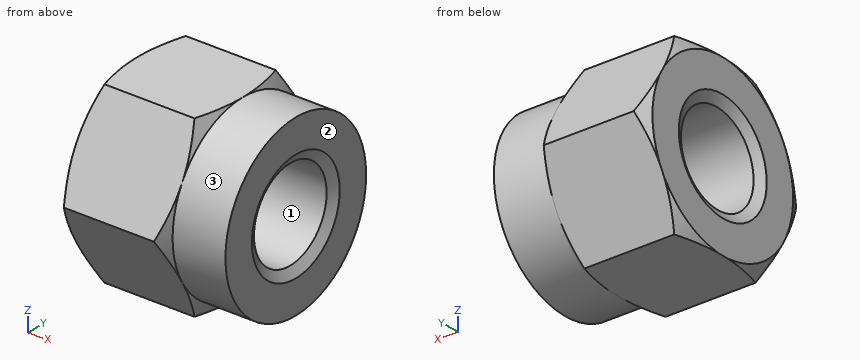
Autodesk Inventor part; units mm, degrees
ref_plane "Work Plane1" through (14.1836, 0, 0) normal (0, 0, 1) x (-1, 0, 0)
ref_plane "YZ Plane" through (0, 0, 0) normal (1, 0, 0) x (0, 1, 0)
ref_plane "XZ Plane" through (0, 0, 0) normal (0, 1, 0) x (-1, 0, 0)
sketch "Sketch1" plane through (0, 0, 0) normal (1, 0, 0) x (0, 1, 0)
  line L0 (2.3094, -4) -> (-2.3094, -4)
  line L1 (-2.3094, -4) -> (-4.6188, 0)
  line L2 (-4.6188, 0) -> (-2.3094, 4)
  line L3 (-2.3094, 4) -> (2.3094, 4)
  line L4 (2.3094, 4) -> (4.6188, 0)
  line L5 (4.6188, 0) -> (2.3094, -4)
  point P0 (0, 0)
  point P1 (0, 0)
  dimension "d0" = 9.2376
extrude "Body" add sketch "Sketch1" along normal blind 4.8
sketch "Sketch2" plane through (4.8, 0, 0) normal (1, 0, 0) x (0, 0, -1)
  circle A0 centre (0, 0) radius 4
  dimension "d7" = 8
extrude "Ring" add sketch "Sketch2" along normal blind 2.4
sketch "Sketch3" plane through (0, 0, 0) normal (0, 0, 1) x (1, 0, 0)
  line L0 (0, 2.3094) -> (0, 4.6188)
  line L1 (0, 4.6188) -> (4.8, 4.6188)
  line L2 (4.8, 2.3094) -> (4.8, 4.6188)
  line L3 (-0.96, 0) -> (5.76, 0)
  line L4 (0, 4) -> (0.3573, 4.6188)
  line L5 (4.4427, 4.6188) -> (4.8, 4)
  dimension "d3" = 30
  dimension "d4" = 30
  dimension "d5" = 8
  dimension "d6" = 8
revolve "Chamfer1" cut sketch "Sketch3" angle 360 about axis through (-10, 0, 0) along (1, 0, 0)
sketch "Sketch4" plane through (0, 0, 0) normal (-1, 0, 0) x (0, 0, 1)
  line L0 (0, -6.4663) -> (0, 6.4663)
  line L1 (-5.6, 0) -> (5.6, 0)
  point P0 (0, 0)
hole "Thread" at (0, 0, 0) direction (1, 0, 0) diameter 4.134 end through all
chamfer "Chamfer2" distance 0.433 angle 30 1 edges at (0, 0, -2.067) measured on face at (0, -3.336, 0.083)
chamfer "Chamfer3" distance 0.433 angle 30 1 edges at (7.2, 0, -2.067) measured on face at (7.2, -0.484, -3.2969)
ref_plane "Work Plane1" through (14.1836, 0, 0) normal (0, 0, 1) x (-1, 0, 0)
equation "\"d0\" = 1.1547 * SW"
equation "\"d1\" = KOH1"
equation "\"d7\" = SD2"
equation "\"d8\" = KOH - KOH1"
equation "\"d3\" = ANG1"
equation "\"d4\" = ANG2"
equation "\"d5\" = SW0"
equation "\"d6\" = SW01"
equation "\"d10\" = -0.5 * GD1 + 0.5 * NND"
equation "\"d46\" = -0.5 * GD1 + 0.5 * NND"
equation "\"d12\" = -0.5 * GD1 + 0.5 * NND"
equation "\"d47\" = -0.5 * GD1 + 0.5 * NND"
equation "\"ANG1\" = 30deg"
equation "\"ANG2\" = 30deg"
equation "\"NND\" = 5"
equation "\"KOH1\" = 4.8"
equation "\"KOH\" = 7.2"
equation "\"SW\" = 8"
equation "\"SW0\" = SW"
equation "\"SW01\" = SW"
equation "\"SD2\" = SW"
equation "\"GUL\" = 0.541266 * PTC"
equation "\"THREADDIA\" = 5"
equation "\"TOA\" = 30deg"
equation "\"PTC\" = 0.8"
equation "\"GAL\" = 0.541266 * PTC"
equation "\"E0\" = 1.155 * SW"
properties part number "ISO 7041 - M5" material "Steel"
Build history of the part. All positions in model axes, mm. Face numbers are marked on the shaded views. Give positions to 0.01 mm unless a question says otherwise; leave off trailing zeros. Write each loop counter-clockwise with the first axis right and the second up, starting at its lowest first coordinate (ties: lowest second). Pieces come first, ordered by that corner, then holes. Notation, with made-up numbers: (8, -36) - (25, -36) arc R20 ccw to (25, -22) - close; hole circle Ø10 at (-38.75, 12). An arc over 180 degrees is marked (long way). Use one line per item in the form item = value. Start each with the question number.
1. Band-saw the part on B-B on x = 5.5. Write the cut outline in (y, z), plus the area to 3 significant figures.
2. Band-saw the part on A-A on x = 4.25. Write the cut outline in (y, z).
3. Drop a flat-ended pin along its axis: pin 1 Ø2 at (x, z) = (2, -2.5) entering from -Y. Give the stop position or say it passes through.
4. Probe line 1 (Z direction, x = 2, y = 0); line 2 (Z direction, x = 4, y = 0.75); line 3 (Y direction, x = 6.5, z = -0.75). List the from-to ranges inside material, lowest first. Write a range as [from, to].
5. Two-plate mould, pull along Y, no slides. Class the marked faces 1, 2 and 3: released by +Y, released by -Y, zero draft, split by the parting line, or undercut.
Conclusion:
q1.outline = circle Ø8 at (0, 0); hole circle Ø4.13 at (0, 0)
q1.area = 36.8 mm²
q2.outline = (-4.62, 0) - (-2.31, -4) - (2.31, -4) - (4.62, 0) - (2.31, 4) - (-2.31, 4) - close; hole circle Ø4.13 at (0, 0)
q3.pin_1 = -3.75
q4.line_1 = [-4, -2.07], [2.07, 4]
q4.line_2 = [-4, -1.93], [1.93, 4]
q4.line_3 = [-3.93, -1.93], [1.93, 3.93]
q5.face_1 = undercut
q5.face_2 = zero draft
q5.face_3 = split by the parting line
